```python
from build123d import *

# Parameters (mm, degrees)
BOSS_EXTRUDE1_DEPTH = 1.5
FILLET1_R           = 50


with BuildPart() as part:
    # Sketch2 → Boss-Extrude1 (new, symmetric)
    with BuildSketch(Plane.XY):
        Polygon((15, 44), (30, 44), (30, 56), (25, 56), (25, 59), (-25, 59), (-25, 56), (-30, 56), (-30, 44), (-15, 44), (-15, -44), (-10, -44), (-10, -47), (10, -47), (10, -44), (15, -44), align=None)
    extrude(amount=BOSS_EXTRUDE1_DEPTH, both=True)

    # Fillet1
    # the kernel refuses this fillet: 50 mm, written as the material it adds along each edge
    with BuildSketch(Plane(origin=(-15, 44, -1.5), x_dir=(0, -1, 0), z_dir=(0, 0, 1))) as fillet1_piece_1:
        with BuildLine():
            CenterArc((35.707142143, -50), FILLET1_R, 90, 45.572995999)
            Line((0, -15), (-0.714142843, -14.3))
            ThreePointArc((-0.714142843, -14.3), (-1, -7.5), (-1, 0))
            Line((-1, 0), (0, 1))
            Line((0, 1), (35.707142143, 1))
            Line((35.707142143, 1), (35.707142143, 0))
        make_face()
    extrude(amount=3)
    with BuildSketch(Plane(origin=(15, 44, 1.5), x_dir=(1, 0, 0), z_dir=(0, 0, -1))) as fillet1_piece_2:
        with BuildLine():
            CenterArc((50, 35.707142143), FILLET1_R, 180, 45.572995999)
            Line((0, 35.707142143), (-1, 35.707142143))
            Line((-1, 35.707142143), (-1, 0))
            Line((-1, 0), (0, -1))
            ThreePointArc((0, -1), (7.5, -1), (14.3, -0.714142843))
            Line((14.3, -0.714142843), (15, 0))
        make_face()
    extrude(amount=3)


solid = part.part
```
The model under review builds one solid part; all positions refer to its coordinate system, in mm. A direction names the side the tool comes from. Give positions to 0.01 mm unless a question says otherwise; leave off trailing zeros. Write each loop counter-clockwise with the first axis right and the second up, starting at its lowest first coordinate (ties: lowest second). Pieces come first, ordered by that corner, then holes.
(1) Consider section C-C, the plane x = -14. Give the boundary of the cut face in (y, z).
(2) For P1, Ø1.5, axis at y = 57.5, z = 0.5, coming from the +X side; P2, Ø0.9, axis at y = 57, z = 0, coming from the -X side; P3, Ø0.9, axis at y = -45.5, z = 0, coming from the -X side; P4, Ø6, axis at x = -17, y = -22.5, coming from the -Z side, all flat-tipped, find the tip position at first contact; note any pin that passes through.
(3) Tool access review of faces 1 (the flat face through (0, 5, -1.5)), 2 (the flat face through (-13, -44, 0)), 3 (the flat face through (-27, 56, 0)), 4 (the flat face through (25, 57, 0)), 5 (the flat face through (12, -44, 0)): name each direction out of +Z, -Z, +X, -X, +Y, -Y from which nothing blocks a thin tool from reaching the whole face with its end or side.
(4) Consider section A-A, the plane z = 0. Give the boundary of the cut face in (x, y), and give its area (3 significant figures).
(5) To check wall thickness, follow L1, parallel to X at y = -33.5, z = 0.25; L2, parallel to Y at x = -14, z = 1.1; L3, parallel to Y at x = -19, z = 0.4. State the ranges of each line that lie inside material, in increasing order.
(6) Consider section B-B, the plane y = 3.5. Give the boundary of the cut face in (x, z), and give its area (3 significant figures).
Returned:
1. outline: (-44, -1.5) - (59, -1.5) - (59, 1.5) - (-44, 1.5) - close
2. P1: stops at x = 25
2. P2: stops at x = -25
2. P3: stops at x = -10
2. P4: stops at z = -1.5
3. face 1: -Z, +X, -X, +Y, -Y
3. face 2: +Z, -Z, -X, -Y
3. face 3: +Z, -Z, -X, +Y
3. face 4: +Z, -Z, +X, +Y
3. face 5: +Z, -Z, +X, -Y
4. outline: (-30, 44) arc R50 cw to (-15, 8.29) - (-15, -44) - (-10, -44) - (-10, -47) - (10, -47) - (10, -44) - (15, -44) - (15, 8.29) arc R50 cw to (30, 44) - (30, 56) - (25, 56) - (25, 59) - (-25, 59) - (-25, 56) - (-30, 56) - close
4. area: 3,900 mm2
5. L1: x = -15 to 15
5. L2: y = -44 to 59
5. L3: y = 27.89 to 59
6. outline: (-15, -1.5) - (15, -1.5) - (15, 1.5) - (-15, 1.5) - close
6. area: 90.0 mm2
